Study the drawing (mm; zero at the part's minimum x, y, z) and answer. Give positions to 0.01 mm unless a question says otherwise; leave off trailing zeros. Loops run counter-clockwise (first coordinate to the right, second up) from the corner with the lowest first, then second, coordinate; pieces in that order, holes last. Notation, with made-up numbers: M -21.5,30 L -2.5,30 A24 cw -2.5,41 Z; hole C -14.5,69 d5. An arc over 180 degrees is marked long. Return JSON: item names as keys, results as strings.
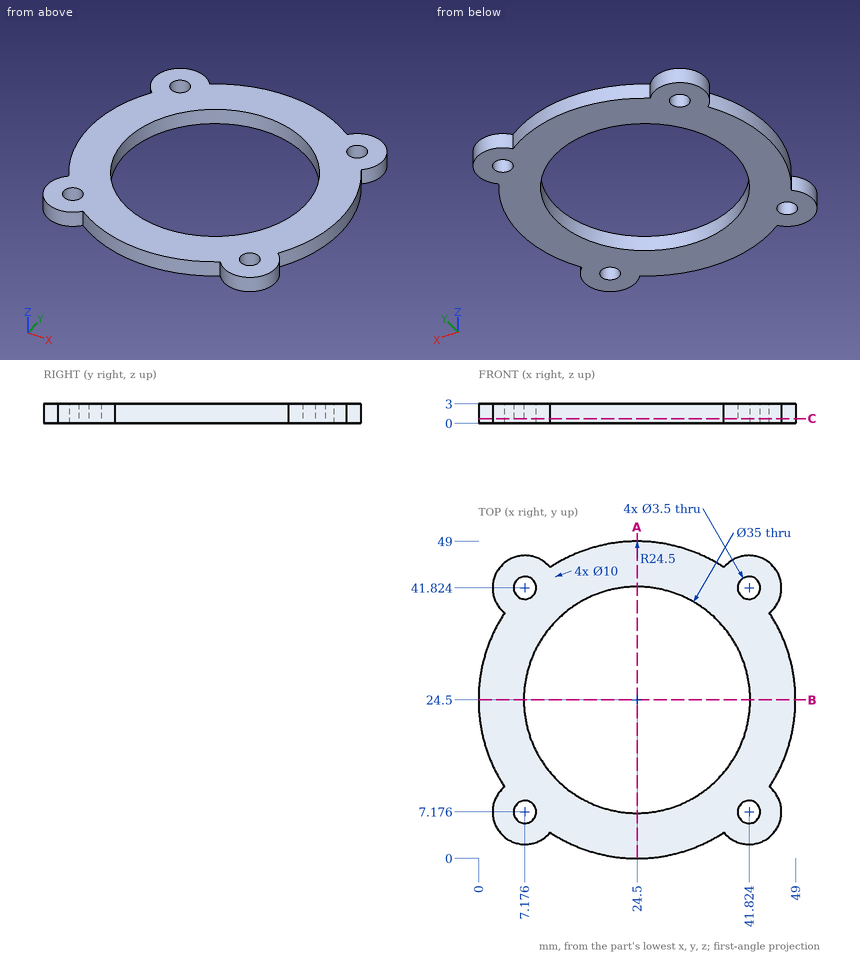
(1) Given pin 1 (21 mm diameter, centred on x = 24.5, y = 24.5, fed in from -Z); pin 2 (1 mm diameter, centred on y = 33.5, z = 1.5, fed in from -X), each flat-ended and moving along its own axis, determine where each tip first touches the part or whether it passes through.
Values follow:
{"pin 1": "through", "pin 2": "x = 1.52"}
(2) Straight lines are drawn through the part: line 1 along Y through (x, z) = (24.5, 2.35); line 2 along X through (y, z) = (3, 2.4) (1 decimal); line 3 along X through (y, z) = (8.5, 1.85) (1 decimal). For each, find the intervals that lie inside material, in ascending order.
Values follow:
{"line 1": "0 to 7, 42 to 49", "line 2": "4.4 to 9.9, 12.8 to 36.2, 39.1 to 44.6", "line 3": "2.4 to 6, 8.3 to 17.4, 31.6 to 40.7, 43 to 46.6"}
(3) The part is cut by section C-C (z = 0.75). Determine the outline of the cut face in (x, y), and give its area (3 significant figures).
Values follow:
{"outline": "M 4.02,11.05 A5 ccw long 11.05,4.02 A24.5 ccw 37.95,4.02 A5 ccw long 44.98,11.05 A24.5 ccw 44.98,37.95 A5 ccw long 37.95,44.98 A24.5 ccw 11.05,44.98 A5 ccw long 4.02,37.95 A24.5 ccw Z; hole C 7.18,7.18 d3.5; hole C 7.18,41.82 d3.5; hole C 24.5,24.5 d35; hole C 41.82,7.18 d3.5; hole C 41.82,41.82 d3.5", "area": "1,050 mm²"}
(4) The part is cut by section A-A (x = 24.5). Determine the outline of the cut face in (y, z).
Values follow:
{"outline": "M 0,0 L 7,0 L 7,3 L 0,3 Z; M 42,0 L 49,0 L 49,3 L 42,3 Z"}
